The listing builds one solid part. Answer for the finished solid, in the listing's coordinates (mm). A direction names the side the tool comes from. Round coordinates to 2 decimals unless told otherwise and drop trailing zeros. Loops run counter-clockwise (first coordinate to the right, second up) from the corner with the lowest first, then second, coordinate; pieces in that order, holes last. Notation, with made-up numbers: M 5.25,7.25 L 13.25,7.25 A19 cw 13.25,17.25 Z; hole C 34,-20.75 d1. An arc over 180 degrees is marked long. Put each result on its own line as item: value. Start each with the question number.
(1) Which of the six approach directions +Z, -Z, +X, -X, +Y, -Y give full straight-line access (tool end or side, diameter ignored) to faces 1 (the face through (-6.23, 3.2, 1.91)), 2 (the face through (5.81, 6.71, -7.58)), 3 (the face through (-20.474, -9.555, -2.688))?
(2) Section A-A, the plane y = 8.25 is taken. Determine the outline of the cut face in (x, z).
(3) Section B-B, the plane y = -3.5 is taken. Determine the outline of the cut face in (x, z).
(4) Flat-ended cylindrical pins translate along their axes: P1, Ø4, axis at y = 5.5, z = -13.5, coming from the -X side; P2, Ø1, axis at x = -0.5, y = 3.5, coming from the -Z side; P3, Ø12, axis at x = 13, y = -8, coming from the -Z side; P4, Ø6, axis at x = 5.5, y = -1, coming from the -Z side. Find the tip coordinate at first contact, or state that the pin passes through.
(5) Straight lines are drawn through the part: line 1 (X direction, y = 5.5, z = 0); line 2 (X direction, y = -0.5, z = 0). For each, find the intervals that lie inside material, in ascending order.
(6) Determine the mould class of faces 4 (the face through (3.905, 0.144, -0.867)), 5 (the face through (-5, -10.3, 0)), 6 (the face through (6.2, 2.95, -1.38)) for opening direction Y: released by +Y, released by -Y, zero draft, split by the parting line, or undercut.
```python
from build123d import *

# Parameters (mm, degrees)
F2_C1_SIZE2 = 0.4
F2_C1_SIZE  = 0.8
F2_C2_SIZE2 = 0.8
F2_C2_SIZE  = 0.4
F2_C3_SIZE2 = 0.8
F2_C3_SIZE  = 0.4
F3_SIZE2    = 0.4
F3_SIZE     = 0.8
F4_SIZE     = 0.4


with BuildPart() as f1:
    # F0 (on Right) → F1 (revolve)
    with BuildSketch(Plane.YZ):
        Polygon((-10.3, 20.65), (-10.3, 4), (10.3, 4), (10.3, 9.55), (3.2, 9.55), (3.2, 6.35), (2.7, 6.35), (2.7, 20.65), (1.2, 20.65), (1.2, 19.1), (-8.8, 19.1), (-8.8, 20.65), align=None)
    revolve(axis=Axis((0, -3.1587743408, 0), (0, -1, 0)))

    # F2: chamfer of 0.4 x 0.8 on 3 edges, made by hand

    # F2_c1
    f2_c1_edges = [f1.edges().sort_by_distance(p)[0] for p in [
        (0, -10.3, -20.65),
    ]]
    f2_c1_side = f1.faces().sort_by_distance((0, -10.3, -20.642))[0]
    chamfer(f2_c1_edges, length=F2_C1_SIZE, length2=F2_C1_SIZE2, reference=f2_c1_side)

    # F2_c2
    f2_c2_edges = [f1.edges().sort_by_distance(p)[0] for p in [
        (0, 2.7, -20.65),
    ]]
    f2_c2_side = f1.faces().sort_by_distance((0, 2.692, -20.65))[0]
    chamfer(f2_c2_edges, length=F2_C2_SIZE, length2=F2_C2_SIZE2, reference=f2_c2_side)

    # F2_c3
    f2_c3_edges = [f1.edges().sort_by_distance(p)[0] for p in [
        (0, 1.2, -20.65),
    ]]
    f2_c3_side = f1.faces().sort_by_distance((0, 1.208, -20.65))[0]
    chamfer(f2_c3_edges, length=F2_C3_SIZE, length2=F2_C3_SIZE2, reference=f2_c3_side)

    # F3
    f3_edges = [f1.edges().sort_by_distance(p)[0] for p in [
        (0, -8.8, -20.65),
    ]]
    chamfer(f3_edges, length=F3_SIZE, length2=F3_SIZE2)

    # F4
    f4_edges = [f1.edges().sort_by_distance(p)[0] for p in [
        (0, 3.2, -9.55),
        (0, 10.3, -9.55),
    ]]
    chamfer(f4_edges, length=F4_SIZE)


solid = f1.part
```
Recorded:
1. face 1: none
1. face 2: +Y
1. face 3: +Y, -Y
2. outline: C 0,0 d19.1; hole C 0,0 d8
3. outline: C 0,0 d38.2; hole C 0,0 d8
4. P1: passes through
4. P2: stops at z = -9.55
4. P3: stops at z = -19.38
4. P4: stops at z = -20.26
5. line 1: x = -9.55 to -4, 4 to 9.55
5. line 2: x = -19.1 to -4, 4 to 19.1
6. face 4: zero draft
6. face 5: released by -Y
6. face 6: undercut
